The model under review builds one solid part; all positions refer to its coordinate system, in mm. A direction names the side the tool comes from. Round coordinates to 2 decimals unless told otherwise and drop trailing zeros. Order: outer loops, then holes, each group sorted by start corner. A loop starts at its lowest first (then second) coordinate and runs counter-clockwise, first axis right, second up.
from build123d import *

# Parameters (mm, degrees)
EXTRUDE_1_DEPTH                  = 10.5
SKETCH_2_W                       = 102.00000000000001
SKETCH_2_H                       = 75.00000000000009
EXTRUDE_2_DEPTH                  = 19.4993693487819
EXTRUDE_3_DEPTH                  = 18.000000000000004
SKETCH_4_W                       = 18.000000000000004
SKETCH_4_H                       = 140
EXTRUDE_4_DEPTH                  = 70.0006306512181
EXTRUDE_START                    = 10.499999999999998
EXTRUDE_5_DEPTH                  = 10.499999999999998
CUT_EXTRUDE_1_REACH              = 194.401
SKETCH_7_W                       = 4.000000000000014
SKETCH_7_H                       = 29.999999999999993
CUT_EXTRUDE_2_DEPTH              = 201.0099997500125
CUT_EXTRUDE_3_DEPTH              = 210.76176963403032
CUT_EXTRUDE_4_DEPTH              = 210.76176963403032
EXTRUDE_6_DEPTH                  = 0.7500000000000007
HOLE_WIZARD_M521_D               = 61.5
EXTRUDE_7_DEPTH                  = 5.749999999999998
HOLE_WIZARD_6_7_6_7_1_AT_2_COUNT = 2
HOLE_WIZARD_6_7_6_7_1_AT_2_PITCH = 45
HOLE_WIZARD_4_0_4_1_AT_2_COUNT   = 2
HOLE_WIZARD_4_0_4_1_AT_2_PITCH   = 49.49747468305833
CHAMFER_1_SIZE                   = 0.9999999999999991
EXTRUDE_START_2                  = -16.249369
SKETCH_28_R                      = 3.35
SKETCH_28_R_2                    = 9.999999999999993
SKETCH_28_R_3                    = 3.350000000000003
EXTRUDE_8_DEPTH                  = 16.249369


with BuildPart() as part:
    # Эскиз1 → Бобышка-Вытянуть1 (new body)
    with BuildSketch(Plane(origin=(29.9993693487819, 0, 0), x_dir=(0, 0, -1), z_dir=(1, 0, 0))):
        with BuildLine():
            Line((14.919229074297327, 90.0005475751909), (0, 90.0005475751909))
            Line((0, 90.0005475751909), (0, 15.0005475751908))
            Line((0, 15.0005475751908), (102.00000000000001, 15.0005475751908))
            Line((102.00000000000001, 15.0005475751908), (85.69382268537409, 20.93551075238141))
            ThreePointArc((85.69382268537409, 20.93551075238141), (74.94644857866616, 27.70982740688085), (67.9664449575318, 38.324768093192546))
            ThreePointArc((67.9664449575318, 38.324768093192546), (24.088528585175357, 46.3477790832992), (14.919229074297327, 90.0005475751909))
        make_face()
    extrude(amount=-EXTRUDE_1_DEPTH)

    # Эскиз2 → Бобышка-Вытянуть2 (add)
    with BuildSketch(Plane.ZY.offset(-19.4993693487819)):
        with Locations((-51.00000000000001, 52.50054757519085)):
            Rectangle(SKETCH_2_W, SKETCH_2_H)
    extrude(amount=EXTRUDE_2_DEPTH)

    # Эскиз3 → Бобышка-Вытянуть3 (add)
    with BuildSketch(Plane.XY):
        Polygon((29.999369348781915, -6.94e-15), (3.47e-15, 15.000547575190799), (0, 124.997494914823), (29.997641385548, 140), (29.999369348781904, 140), align=None)
    extrude(amount=EXTRUDE_3_DEPTH)

    # Эскиз4 → Бобышка-Вытянуть4 (add)
    with BuildSketch(Plane(origin=(29.9993693487819, 0, 0), x_dir=(0, 0, -1), z_dir=(1, 0, 0))):
        with Locations((-9.000000000000002, 70)):
            Rectangle(SKETCH_4_W, SKETCH_4_H)
    extrude(amount=EXTRUDE_4_DEPTH)

    # Эскиз5 → Бобышка-Вытянуть5 (add)
    with BuildSketch(Plane(origin=(19.4993693487819, 0, 0), x_dir=(0, 0, -1), z_dir=(1, 0, 0)).offset(EXTRUDE_START)):
        with BuildLine():
            Line((89.08077092570272, 90.0005475751909), (102.00000000000001, 90.0005475751909))
            Line((102.00000000000001, 90.0005475751909), (102.00000000000001, 23.000547575190808))
            Line((102.00000000000001, 23.000547575190808), (91.92678266011816, 26.666898850201964))
            ThreePointArc((91.92678266011816, 26.666898850201964), (81.8910585435448, 32.765618882150974), (74.9654117449494, 42.24958224106233))
            ThreePointArc((74.9654117449494, 42.24958224106233), (90.35915387380979, 63.660894475956894), (89.08077092570272, 90.0005475751909))
        make_face()
    extrude(amount=-EXTRUDE_5_DEPTH)

    # Эскиз6 → Вырез-Вытянуть1 (cut, up to next)
    with BuildSketch(Plane(origin=(16.2493693487819, 0, 0), x_dir=(0, -1, 0), z_dir=(-1, 0, 0)), mode=Mode.PRIVATE) as cut_extrude_1_sk1:
        with BuildLine():
            Line((-90.0005475751909, -14.919229074297327), (-90.0005475751909, -89.08077092570272))
            ThreePointArc((-90.0005475751909, -89.08077092570272), (-34.999999999999936, -52), (-90.0005475751909, -14.919229074297327))
        make_face()
    cut_extrude_1_tool1 = extrude(cut_extrude_1_sk1.sketch, amount=-CUT_EXTRUDE_1_REACH, mode=Mode.PRIVATE) & part.part
    add(cut_extrude_1_tool1.solids().sort_by_distance((16.249369, 65.774947, -52))[0], mode=Mode.SUBTRACT)

    # Эскиз7 → Вырез-Вытянуть2 (cut, through all)
    with BuildSketch(Plane.ZY):
        with Locations((-100, 75.0005475751909)):
            Rectangle(SKETCH_7_W, SKETCH_7_H)
    extrude(amount=-CUT_EXTRUDE_2_DEPTH, mode=Mode.SUBTRACT)

    # Эскиз8 → Вырез-Вытянуть3 (cut, through all)
    with BuildSketch(Plane.XY.offset(18.000000000000004)):
        with BuildLine():
            Line((64, 140), (45.999999999999986, 140))
            Line((45.999999999999986, 140), (46, 120))
            ThreePointArc((46, 120), (55, 111), (64, 120))
            Line((64, 120), (64, 140))
        make_face()
    extrude(amount=-CUT_EXTRUDE_3_DEPTH, mode=Mode.SUBTRACT)

    # Эскиз9 → Вырез-Вытянуть4 (cut, through all)
    with BuildSketch(Plane.XY.offset(18.000000000000004)):
        with BuildLine():
            Line((46.00000000000001, 0), (64, 0))
            Line((64, 0), (64, 20.000000000000004))
            ThreePointArc((64, 20.000000000000004), (55, 29), (45.999999999999986, 20.000000000000004))
            Line((45.999999999999986, 20.000000000000004), (46.00000000000001, 0))
        make_face()
    extrude(amount=-CUT_EXTRUDE_4_DEPTH, mode=Mode.SUBTRACT)

    # Эскиз10 → Бобышка-Вытянуть6 (add)
    with BuildSketch(Plane(origin=(16.2493693487819, 0, 0), x_dir=(0, 0, -1), z_dir=(1, 0, 0))):
        with BuildLine():
            Line((15.729542704227807, 90.0005475751909), (88.27045729577222, 90.00054757519085))
            ThreePointArc((88.27045729577222, 90.00054757519085), (51.999999999999986, 35.75000000000001), (15.729542704227807, 90.0005475751909))
        make_face()
    extrude(amount=EXTRUDE_6_DEPTH)

    # Отверстие с зазором M521 (through all)
    with Locations(Plane(origin=(16.999369348781904, 0, 0), x_dir=(0, 0, -1), z_dir=(1, 0, 0))):
        with Locations((52, 75)):
            Hole(HOLE_WIZARD_M521_D / 2)

    # Эскиз14 → Отверстие1 (revolve, cut)
    with BuildSketch(Plane(origin=(29.9993693487819, 27.0005475751908, -62), x_dir=(0, 0, -1), z_dir=(0, 1, 0))):
        Polygon((0, 0), (0, 29.9993693487819), (3.1869530848864884, 29.9993693487819), (3.186953084886492, -8.3e-16), align=None)
    revolve(axis=Axis((-80.0006306512181, 27.0005475751908, -62), (1, 0, 0)), mode=Mode.SUBTRACT)

    # Эскиз20 → Диаметр отверстия Ø4.0 (4)1 (revolve, cut)
    with BuildSketch(Plane(origin=(16.999369348781904, 75, -17), x_dir=(0, 0, -1), z_dir=(0, 1, 0))):
        Polygon((0, 0), (-4.16e-15, 16.999369348781904), (1.9999999999999978, 16.999369348781904), (1.9999999999999896, -1.31e-15), align=None)
    hole_wizard_4_0_4_1 = revolve(axis=Axis((23.349369348781895, 75, -17), (-1, 0, 0)), mode=Mode.SUBTRACT)

    # Диаметр отверстия Ø4.0 (4)1 at 2: Диаметр отверстия Ø4.0 (4)1 ×2
    with Locations(*[Vector(0, -0.7071067811865475, -0.7071067811865477) * (i * HOLE_WIZARD_4_0_4_1_AT_2_PITCH) for i in range(1, HOLE_WIZARD_4_0_4_1_AT_2_COUNT)]):
        add(hole_wizard_4_0_4_1, mode=Mode.SUBTRACT)

    # Эскиз22 → Диаметр отверстия Ø6.0 (6)1 (revolve, cut)
    with BuildSketch(Plane(origin=(29.9993693487819, 40.0005475751908, -90), x_dir=(0, 0, -1), z_dir=(0, 1, 0))):
        Polygon((0, 0), (-7.35e-15, 30.000369348781906), (2.9999999999999867, 30.000369348781906), (2.9999999999999907, -1.19e-15), align=None)
    revolve(axis=Axis((36.34936934878189, 40.0005475751908, -90), (-1, 0, 0)), mode=Mode.SUBTRACT)


with BuildPart() as body_2:
    # Эскиз13 → Бобышка-Вытянуть7 (new body)
    with BuildSketch(Plane(origin=(16.2493693487819, 0, 0), x_dir=(0, -1, 0), z_dir=(-1, 0, 0))):
        with BuildLine():
            Line((-90.0005475751909, -26.01955403684463), (-90.0005475751909, -77.98044596315543))
            ThreePointArc((-90.0005475751909, -77.98044596315543), (-44.99999999999993, -51.99999999999999), (-90.0005475751909, -26.01955403684463))
        make_face()
    extrude(amount=-EXTRUDE_7_DEPTH)

    # Эскиз16 → Диаметр отверстия Ø6.7 (6.7)1 (revolve, cut)
    with BuildSketch(Plane(origin=(21.9993693487819, 75, -74.5), x_dir=(0, 0, -1), z_dir=(0, 1, 0))):
        Polygon((0, 0), (-1.41e-15, 5.749999999999998), (3.3500000000000045, 5.749999999999998), (3.3499999999999934, -1.15e-15), align=None)
    hole_wizard_6_7_6_7_1 = revolve(axis=Axis((28.34936934878189, 75, -74.5), (-1, 0, 0)), mode=Mode.SUBTRACT)

    # Диаметр отверстия Ø6.7 (6.7)1 at 2: Диаметр отверстия Ø6.7 (6.7)1 ×2
    with Locations(*[(0, 0, i * HOLE_WIZARD_6_7_6_7_1_AT_2_PITCH) for i in range(1, HOLE_WIZARD_6_7_6_7_1_AT_2_COUNT)]):
        add(hole_wizard_6_7_6_7_1, mode=Mode.SUBTRACT)

    # Эскиз18 → Диаметр отверстия Ø20.0 (20)1 (revolve, cut)
    with BuildSketch(Plane(origin=(21.9993693487819, 75, -52.00000000000001), x_dir=(0, 0, -1), z_dir=(0, 1, 0))):
        Polygon((0, 0), (-1.41e-15, 5.7510000000000066), (9.99999999999999, 5.7510000000000066), (9.99999999999999, -3.3e-16), align=None)
    revolve(axis=Axis((28.34936934878189, 75, -52.00000000000001), (-1, 0, 0)), mode=Mode.SUBTRACT)


with BuildPart() as hole_wizard_5_0_5_1_tool:
    # Эскиз24 → Диаметр отверстия Ø5.0 (5)1 (revolve)
    with BuildSketch(Plane(origin=(23, 75.0005475751909, -98), x_dir=(0, 1, 0), z_dir=(1, 0, 0))):
        Polygon((0, 0), (-1.127e-14, 45.999999999999986), (2.499999999999981, 45.999999999999986), (2.4999999999999867, -1.25e-15), align=None)
    revolve(axis=Axis((23, 75.0005475751909, -104.35), (0, 0, 1)))


with BuildPart() as part_1:
    add(part.part)

    # Диаметр отверстия Ø5.0 (5)1: cut by hole_wizard_5_0_5_1_tool
    add(hole_wizard_5_0_5_1_tool.part, mode=Mode.SUBTRACT)

    # Эскиз26 → Отверстие с зазором M61 (revolve, cut)
    with BuildSketch(Plane(origin=(15.8866729980809, 33.128633292951, -102.00000000000001), x_dir=(0, 1, 0), z_dir=(1, 0, 0))):
        Polygon((0, 0), (-1.47e-15, 5.999999999999993), (3.2357711959407984, 6.000000000000005), (3.2357711959408, -1.16e-15), align=None)
    revolve(axis=Axis((15.8866729980809, 33.128633292951, -108.35000000000001), (0, 0, 1)), mode=Mode.SUBTRACT)


with BuildPart() as body_2_1:
    add(body_2.part)

    # Диаметр отверстия Ø5.0 (5)1: cut by hole_wizard_5_0_5_1_tool
    add(hole_wizard_5_0_5_1_tool.part, mode=Mode.SUBTRACT)

    # Фаска1
    chamfer_1_edges = [body_2_1.edges().sort_by_distance(p)[0] for p in [
        (21.9993693487819, 74.99943746278025, -42.00000001582242),
    ]]
    chamfer(chamfer_1_edges, length=CHAMFER_1_SIZE)


with BuildPart() as extrude_8_tool:
    # Эскиз28 → Бобышка-Вытянуть8 (new body)
    with BuildSketch(Plane.ZY.offset(EXTRUDE_START_2)):
        with BuildLine():
            Line((-78.84298926059529, 90.0005475751909), (-25.157010739404722, 90.0005475751909))
            ThreePointArc((-25.157010739404722, 90.0005475751909), (-52.000000000000014, 44.250000000000014), (-78.84298926059529, 90.0005475751909))
        make_face()
        with Locations(Location((-29.500000000000004, 75, 0), (0, 0, 180))):
            Circle(SKETCH_28_R, mode=Mode.SUBTRACT)
        with Locations(Location((-52.00000000000001, 75, 0), (0, 0, 188.618876561))):
            Circle(SKETCH_28_R_2, mode=Mode.SUBTRACT)
        with Locations(Location((-74.5, 75, 0), (0, 0, 223.135094042))):
            Circle(SKETCH_28_R_3, mode=Mode.SUBTRACT)
    extrude(amount=EXTRUDE_8_DEPTH)


with BuildPart() as part_2:
    add(part_1.part)


with BuildPart() as part_3:
    # Бобышка-Вытянуть8: joined with extrude_8_tool
    add(part_2.part.fuse(extrude_8_tool.part, body_2_1.part, tol=0.00001))


solid = part_3.part
(1) To check wall thickness, follow L1, parallel to Z at x = 10, y = 75; L2, parallel to Y at x = 11, z = -52; L3, parallel to Y at x = 7.25, z = -29.5. State the ranges of each line that lie inside material, in increasing order.
(2) We need section D-D (y = 12.5). Give the boundary of the cut face in (x, z), and give its area (3 significant figures).
(3) Tool access review of faces 1 (the cylindrical face through (20.5, 75, -67)), 2 (the cylindrical face through (11.15, 71.68, -29.06)), 3 (the flat face through (15, 60.001, -100)), 4 (the cylindrical face through (23.028, 35.015, -53.095)): name each direction out of +Z, -Z, +X, -X, +Y, -Y from which nothing blocks a thin tool from reaching the whole face with its end or side.
(4) We need section B-B (y = 123). Give the boundary of the cut face in (x, z).
(5) We need section A-A (z = -52). Give the boundary of the cut face in (x, y).
(6) We need section C-C (x = 86). Give the boundary of the cut face in (y, z).
(7) Clearance check with flat-ended pins moving along their axes: P1, Ø4, axis at x = 38, y = 105, coming from the -Z side; P2, Ø22.5, axis at y = 78.5, z = -37.5, coming from the +X side; P3, Ø9, axis at y = 133.5, z = 10, coming from the -X side; P4, Ø5, axis at y = 27, z = -62, coming from the +X side. State where each tip first meets the part, or that it passes through.
(8) The part is to be moulded in two halves that separate along X. For faces 5 (the flat face through (46, 130, 9)), 6 (the flat face through (15, 38, -102)), 7 (the conical face through (21.16, 74.57, -41.85)), say which applies: pulls with the +X half, pulls with the -X half, needs draft (parallel to the pull), parting line crosses it, or undercut.
Verdict:
1. L1: z = -98 to -77.85, -71.15 to -62, -42 to -32.85, -26.15 to -19, -15 to 18
1. L2: y = 15 to 38, 42 to 65, 85 to 90
1. L3: y = 15 to 71.65, 78.35 to 90
2. outline: (5, 0) - (46, 0) - (46, 18) - (5, 18) - close; (64, 0) - (100, 0) - (100, 18) - (64, 18) - close
2. area: 1,390 mm2
3. face 1: -Z, +X
3. face 2: +X, -X
3. face 3: -Z, +X, -X, +Y
3. face 4: +X
4. outline: (0, 0) - (46, 0) - (46, 18) - (0, 18) - close; (64, 0) - (100, 0) - (100, 18) - (64, 18) - close
5. outline: (0, 15) - (30, 15) - (30, 35) - (16.25, 35) - (16.25, 35.75) - (17, 35.75) - (17, 38) - (0, 38) - close; (0, 42) - (17, 42) - (17, 44.25) - (16.25, 44.25) - (16.25, 45) - (22, 45) - (22, 64) - (21, 65) - (0, 65) - close; (0, 85) - (21, 85) - (22, 86) - (22, 90) - (0, 90) - close
6. outline: (0, 0) - (140, 0) - (140, 18) - (0, 18) - close
7. P1: stops at z = 0
7. P2: stops at x = 22
7. P3: stops at x = 8
7. P4: passes through
8. face 5: undercut
8. face 6: needs draft
8. face 7: pulls with the +X half
